from build123d import *

# Parameters (mm, degrees)
SKETCH_1_R      = 5.05
SKETCH_1_R_2    = 1.55
EXTRUDE_1_DEPTH = 2


with BuildPart() as part:
    # 草图1 → 凸台-拉伸1 (new body)
    with BuildSketch(Plane.XY):
        with BuildLine():
            Line((-23.086792761, -14), (-43.086792761, -14))
            Line((-43.086792761, -14), (-47.086792761, -14))
            Line((-47.086792761, -14), (-47.086792761, -8))
            Line((-47.086792761, -8), (-43.086792761, -8))
            Line((-43.086792761, -8), (-43.086792761, -2.05))
            Line((-43.086792761, -2.05), (-39.086792761, -2.05))
            Line((-39.086792761, -2.05), (-39.086792761, -3.741370628))
            Line((-39.086792761, -3.741370628), (-35.886792761, -3.741370628))
            Line((-35.886792761, -3.741370628), (-35.886792761, -2.05))
            Line((-35.886792761, -2.05), (-32.686792761, -2.05))
            Line((-32.686792761, -2.05), (-32.686792761, 2.05))
            Line((-32.686792761, 2.05), (-35.886792761, 2.05))
            Line((-35.886792761, 2.05), (-35.886792761, 3.741370628))
            Line((-35.886792761, 3.741370628), (-39.086792761, 3.741370628))
            Line((-39.086792761, 3.741370628), (-39.086792761, 2.05))
            Line((-39.086792761, 2.05), (-43.086792761, 2.05))
            Line((-43.086792761, 2.05), (-43.086792761, 8))
            Line((-43.086792761, 8), (-47.086792761, 8))
            Line((-47.086792761, 8), (-47.086792761, 14))
            Line((-47.086792761, 14), (-43.086792761, 14))
            Line((-43.086792761, 14), (-23.086792761, 14))
            ThreePointArc((-23.086792761, 14), (22.184698295, 15.389579642), (5.027449154, -26.527810973))
            ThreePointArc((5.027449154, -26.527810973), (0, -18.175825951), (-5.027449154, -26.527810973))
            ThreePointArc((-5.027449154, -26.527810973), (-15.389579642, -22.184698295), (-23.086792761, -14))
        make_face()
        Circle(SKETCH_1_R, mode=Mode.SUBTRACT)
        with Locations((-9.899494937, -9.899494937)):
            Circle(SKETCH_1_R_2, mode=Mode.SUBTRACT)
        with Locations((-9.899494937, 9.899494937)):
            Circle(SKETCH_1_R_2, mode=Mode.SUBTRACT)
        with Locations((9.899494937, 9.899494937)):
            Circle(SKETCH_1_R_2, mode=Mode.SUBTRACT)
        with Locations((9.899494937, -9.899494937)):
            Circle(SKETCH_1_R_2, mode=Mode.SUBTRACT)
    extrude(amount=EXTRUDE_1_DEPTH)


solid = part.part
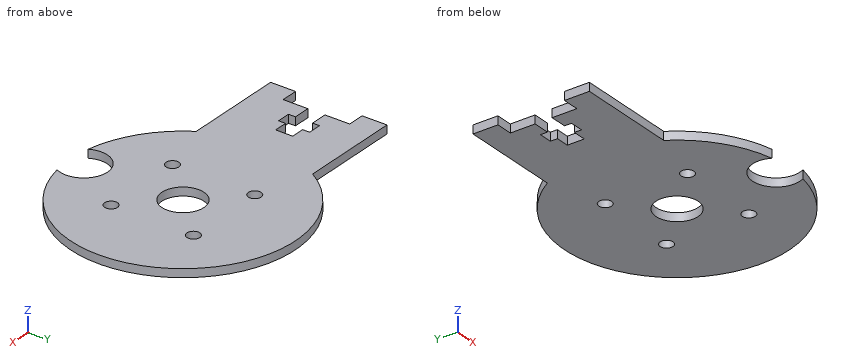
Read the model definition and answer for the solid it produces. Units are mm, in the model's axes. Round coordinates to 2 decimals unless told otherwise and drop trailing zeros. Write each loop counter-clockwise with the first axis right and the second up, starting at its lowest first coordinate (ties: lowest second). Pieces come first, ordered by that corner, then holes.
1. The part is cut by section C-C, the plane z = 1.5. Determine the outline of the cut face in (x, y), then the cut area to 3 significant figures.
2. Straight lines are drawn through the part: L1, parallel to X at y = 3, z = 0.8; L2, parallel to Y at x = -10, z = 0.4; L3, parallel to X at y = 9, z = 1.85. For each, find the intervals that lie inside material, in ascending order.
3. The part is cut by section B-B, the plane x = 0. Determine the outline of the cut face in (y, z), then the cut area to 3 significant figures.
4. The part is cut by section D-D, the plane y = 21.5. Determine the outline of the cut face in (x, z), then the cut area to 3 significant figures.
5. Given pin 1 Ø0.6 at (y, z) = (-0.5, 1) entering from -X; pin 2 Ø1 at (x, z) = (-23, 1) entering from -Y; pin 3 Ø1 at (x, z) = (-41.5, 1.5) entering from -Y, each flat-ended and moving along its own axis, determine where each tip first touches the part or whether it passes through.
6. The part is cut by section A-A, the plane y = 0. Determine the outline of the cut face in (x, z).
Values:
1. outline: (-47.09, -14) - (-23.09, -14) arc R27 ccw to (-5.03, -26.53) arc R5.69 cw (long way) to (5.03, -26.53) arc R27 ccw (long way) to (-23.09, 14) - (-47.09, 14) - (-47.09, 8) - (-43.09, 8) - (-43.09, 2.05) - (-39.09, 2.05) - (-39.09, 3.74) - (-35.89, 3.74) - (-35.89, 2.05) - (-32.69, 2.05) - (-32.69, -2.05) - (-35.89, -2.05) - (-35.89, -3.74) - (-39.09, -3.74) - (-39.09, -2.05) - (-43.09, -2.05) - (-43.09, -8) - (-47.09, -8) - close; hole circle Ø3.1 at (-9.9, -9.9); hole circle Ø3.1 at (-9.9, 9.9); hole circle Ø10.1 at (0, 0); hole circle Ø3.1 at (9.9, -9.9); hole circle Ø3.1 at (9.9, 9.9)
1. area: 2,580 mm2
2. L1: x = -43.09 to -39.09, -35.89 to -4.06, 4.06 to 26.83
2. L2: y = -25.08 to -11.45, -8.35 to 8.35, 11.45 to 25.08
2. L3: x = -47.09 to -11.16, -8.64 to 8.64, 11.16 to 25.46
3. outline: (-18.18, 0) - (-5.05, 0) - (-5.05, 2) - (-18.18, 2) - close; (5.05, 0) - (27, 0) - (27, 2) - (5.05, 2) - close
3. area: 70.2 mm2
4. outline: (-16.33, 0) - (16.33, 0) - (16.33, 2) - (-16.33, 2) - close
4. area: 65.3 mm2
5. pin 1: stops at x = -32.69
5. pin 2: stops at y = -14.92
5. pin 3: stops at y = -14
6. outline: (-32.69, 0) - (-5.05, 0) - (-5.05, 2) - (-32.69, 2) - close; (5.05, 0) - (27, 0) - (27, 2) - (5.05, 2) - close
